Solid Edge part; units mm, degrees
sketch "Sketch1" plane through (0, 0, 0) normal (0, 0, 1) x (1, 0, 0)
  line L0 (-23.7, -18) -> (23.7, -18)
  arc A0 (23.7, -18) -> (27.7, -14) centre (23.7, -14) ccw
  line L1 (27.7, -14) -> (27.7, 14)
  arc A1 (23.7, 18) -> (27.7, 14) centre (23.7, 14) cw
  line L2 (23.7, 18) -> (-23.7, 18)
  arc A2 (-23.7, 18) -> (-27.7, 14) centre (-23.7, 14) ccw
  line L3 (-27.7, 0) -> (-27.7, 14)
  line L4 (-27.7, 0) -> (-27.7, -14)
  arc A3 (-27.7, -14) -> (-23.7, -18) centre (-23.7, -14) ccw
  line L5 (-24.85, -15.15) -> (26.85, -15.15)
  line L6 (26.85, -15.15) -> (26.85, 15.15)
  line L7 (-24.85, 15.15) -> (26.85, 15.15)
  line L8 (-24.85, -15.15) -> (-24.85, 15.15)
extrude "Protrusion1" add sketch "Sketch1" along normal blind 1.2
sketch "Sketch2" plane through (0, 0, 1.2) normal (0, 0, 1) x (1, 0, 0)
  line L0 (-25.1, 15.15) -> (-24.975, -15.15)
  line L1 (-24.975, -15.15) -> (-24.975, -15.35)
  line L2 (-24.975, -15.35) -> (27.05, -15.35)
  line L3 (27.05, -15.35) -> (27.05, -15.15)
  line L4 (27.05, 15.15) -> (27.05, -15.15)
  line L5 (27.05, 15.15) -> (27.05, 15.35)
  line L6 (27.05, 15.35) -> (-25.1, 15.35)
  line L7 (-25.1, 15.35) -> (-25.1, 15.15)
extrude "Wyciągnięcie_2" add sketch "Sketch2" against normal blind 3.45
sketch "Sketch3" plane through (0, 0, 1.2) normal (0, 0, 1) x (-1, 0, 0)
  circle A0 centre (-20.1126, 11.4835) radius 2.95
  circle A1 centre (20.1126, 11.4835) radius 2.95
  circle A2 centre (20.1126, -11.4835) radius 2.95
  circle A3 centre (-20.1126, -11.4835) radius 2.95
extrude "Wycięcie_1" cut sketch "Sketch3" against normal blind 2.7
sketch "Sketch4" plane through (0, 0, 1.2) normal (0, 0, 1) x (-1, 0, 0)
  line L0 (-24.5, -18) -> (24.1, -18)
  arc A0 (27.7, -14.4) -> (24.1, -18) centre (24.1, -14.4) cw
  line L1 (27.7, -14.4) -> (27.7, 14.5)
  arc A1 (24.2, 18) -> (27.7, 14.5) centre (24.2, 14.5) cw
  line L2 (24.2, 18) -> (-24.7, 18)
  arc A2 (-24.7, 18) -> (-27.7, 15) centre (-24.7, 15) ccw
  line L3 (-27.7, 15) -> (-27.7, -14.8)
  arc A3 (-27.7, -14.8) -> (-24.5, -18) centre (-24.5, -14.8) ccw
extrude "Wyciągnięcie_3" add sketch "Sketch4" along normal blind 0.4
Could you check a few things on this model? Use its own coordinates, in mm. A direction names the side the tool comes from. Give positions to 0.01 mm unless a question says otherwise; leave off trailing zeros. Write each loop counter-clockwise with the first axis right and the second up, starting at its lowest first coordinate (ties: lowest second). Pieces come first, ordered by that corner, then holes. Notation, with made-up numbers: (-16.75, 9.25) -> (-7.75, 9.25) arc R18 ccw to (-7.75, 44.25) -> close; hole circle Ø6 at (75, -32). An arc over 180 degrees is marked (long way). Answer as CSV lines item,"result". Start each with the question number.
(1) If we mould it in two halves opening along Y, with no side actions, what happens to faces 6 (the face through (1, 18, 1)), 7 (the face through (20, -11, 1.2)), 8 (the face through (26.6, -17, 1.2))? For each: +Y half, -Y half, draft (parallel to the pull), parting line (faces both ways), or undercut.
(2) If we section it at A-A, the plane x = -3: Write out the boundary of the cut face in (y, z), and give its area (3 significant figures).
(3) If we section it at B-B, the plane x = -19: Write out the boundary of the cut face in (y, z), and give its area (3 significant figures).
(4) Which directions (+Z, -Z, +X, -X, +Y, -Y) give clear straight access to the entire face, cutting with the end or side of a thin tool? Please do faces 1 (the face through (-20, -11, 1.2)), 2 (the face through (26.497, 16.859, 0.592)), 3 (the face through (-26.559, 16.797, 0.592)), 4 (the face through (1, -15.35, -1)), 5 (the face through (-26.497, -16.859, 0.592)).
(5) If we section it at D-D, the plane y = -1.5: Write out the boundary of the cut face in (x, z).
(6) Please list where these lines run through material, in increasing order: line 1 (X direction, y = 11, z = 0.85); line 2 (Y direction, x = 20, z = -0.15); line 3 (X direction, y = -11, z = -0.7).
(7) If we section it at C-C, the plane z = -0.85: Give the number of separate pieces and of enclosed holes in the cut face, and give its area (3 significant figures).
(8) I'm going to push flat-ended pins straight in: pin 1 Ø1.8 at (y, z) = (-5.5, -1) entering from +X; pin 2 Ø1 at (y, z) = (-8.5, -1) entering from -X; pin 3 Ø3 at (x, y) = (-25, 15.5) entering from -Z. Where does each tip first touch, or does it pass through?
Answer list:
1,face 6,"+Y half"
1,face 7,"undercut"
1,face 8,"draft"
2,outline,"(-18, 0) -> (-15.35, 0) -> (-15.35, -2.25) -> (15.35, -2.25) -> (15.35, 0) -> (18, 0) -> (18, 1.6) -> (-18, 1.6) -> close"
2,area,"127 mm^2"
3,outline,"(-18, 0) -> (-15.35, 0) -> (-15.35, -2.25) -> (15.35, -2.25) -> (15.35, 0) -> (18, 0) -> (18, 1.6) -> (-18, 1.6) -> close; hole (-14.22, -1.5) -> (-8.75, -1.5) -> (-8.75, 1.2) -> (-14.22, 1.2) -> close; hole (8.75, -1.5) -> (14.22, -1.5) -> (14.22, 1.2) -> (8.75, 1.2) -> close"
3,area,"97.2 mm^2"
4,face 1,"none"
4,face 2,"-Z, +X, +Y"
4,face 3,"-Z, -X, +Y"
4,face 4,"-Z, +X, -X, -Y"
4,face 5,"-Z, -X, -Y"
5,outline,"(-27.7, 0) -> (-25.03, 0) -> (-25.03, -2.25) -> (27.05, -2.25) -> (27.05, 0) -> (27.7, 0) -> (27.7, 1.6) -> (-27.7, 1.6) -> close"
6,line 1,"-27.7 to -23.02, -17.2 to 17.2, 23.02 to 27.7"
6,line 2,"-15.35 to -14.43, -8.54 to 8.54, 14.43 to 15.35"
6,line 3,"-24.99 to -23.02, -17.2 to 17.2, 23.02 to 27.05"
7,separate pieces,"1"
7,enclosed holes,"4"
7,area,"1,490 mm^2"
8,pin 1,"x = 27.05"
8,pin 2,"x = -25"
8,pin 3,"z = -2.25"
